Autodesk Inventor part; units mm, degrees
ref_plane "YZ Plane" through (0, 0, 0) normal (1, 0, 0) x (0, 1, 0)
ref_plane "XZ Plane" through (0, 0, 0) normal (0, 1, 0) x (-1, 0, 0)
ref_plane "XY Plane" through (0, 0, 0) normal (0, 0, 1) x (1, 0, 0)
sketch "Esquisse6" plane through (20, 29, 11.5) normal (-1, 0, 0) x (0, 0, 1)
  line L0 (0, -22) -> (-23, -22) construction
  line L1 (-23, -30.3566) -> (-23, -22) construction
  line L2 (0, -30.3566) -> (-23, -30.3566) construction
  line L3 (0, -30.3566) -> (0, -22) construction
  line L4 (-23, 0) -> (0, 0) construction
  line L5 (0, 8.3566) -> (0, 0) construction
  line L6 (-23, 8.3566) -> (0, 8.3566) construction
  line L7 (-23, 8.3566) -> (-23, 0) construction
  line L8 (-23, 8.3566) -> (-23, 0) construction
  line L9 (0, 8.3566) -> (-23, 8.3566) construction
  line L10 (0, 8.3566) -> (0, 0) construction
  line L11 (0, 8.3566) -> (0, 0) construction
  line L12 (-23, -30.3566) -> (-22, -27.6783)
  line L13 (-22, -27.6783) -> (-21, -27.6783)
  line L14 (-21, -27.6783) -> (-21, -24.6783)
  line L15 (-21, -24.6783) -> (-22, -24.6783)
  line L16 (-22, -24.6783) -> (-23, -22)
  line L17 (-23, -30.3566) -> (-23, -22) construction
  line L18 (-23, -26.1783) -> (-21, -26.1783) construction
  line L19 (-23, -22) -> (-23, -30.3566)
  line L20 (-23, -30.3566) -> (0, -30.3566)
  line L21 (-11.5, -22) -> (-11.5, -30.3566) construction
  line L22 (-23, -22) -> (0, -22) construction
  line L23 (0, -30.3566) -> (0, -22) construction
  line L24 (-23, -30.3566) -> (0, -30.3566) construction
  line L25 (0, -30.3566) -> (-1, -27.6783)
  line L26 (-1, -27.6783) -> (-2, -27.6783)
  line L27 (-2, -27.6783) -> (-2, -24.6783)
  line L28 (-2, -24.6783) -> (-1, -24.6783)
  line L29 (-1, -24.6783) -> (0, -22)
  line L30 (0, -30.3566) -> (0, -22) construction
  line L31 (0, -26.1783) -> (-2, -26.1783) construction
  line L32 (0, -22) -> (0, -30.3566)
  line L33 (0, -30.3566) -> (-23, -30.3566)
  dimension "d31" = 1
  dimension "d32" = 1
  dimension "d33" = 3
sketch "Esquisse1" plane through (0, 0, 0) normal (0, 1, 0) x (-1, 0, 0)
  arc A0 (0, -11.5) -> (0, 11.5) centre (0, 0) ccw
  line L0 (0, 11.5) -> (-20, 11.5)
  line L1 (-20, 11.5) -> (-20, -11.5)
  line L2 (-20, -11.5) -> (0, -11.5)
  dimension "d0" = 23
  dimension "d1" = 20
  dimension "d2" = 11.5
extrude "Plaque1" add sketch "Esquisse1" along normal blind 3
sketch "Esquisse2" plane through (0, 0, 0) normal (0, -1, 0) x (1, 0, 0)
  arc A0 (0, 11.5) -> (0, -11.5) centre (0, 0) ccw construction
  line L0 (0, 0) -> (-6, 0) construction
  point P0 (0, 6)
  point P1 (0, -6)
  point P2 (6, 0)
  dimension "d6" = 360
  dimension "d8" = 6
hole "Perçage1" at (0, 0, 0) at (0, 0, 6) at (-6, 0, 0) at (0, 0, -6) at (6, 0, 0) direction (0, 1, 0) diameter 4.05 end through all counterbore diameter 5.5 counterbore depth 1
ref_plane "Plan de construction1" through (0, 18, 0) normal (0, 1, 0) x (1, 0, 0)
mirror "Symétrie1" about plane through (0, 18, 0) normal (0, 1, 0)
sketch "Esquisse3" plane through (20, 0, 11.5) normal (1, 0, 0) x (0, 0, -1)
  line L0 (23, 3) -> (0, 3)
  line L1 (0, 0) -> (0, 3)
  line L2 (23, 0) -> (0, 0)
  line L3 (23, 0) -> (23, 3)
  line L4 (23, 33) -> (0, 33)
  line L5 (23, 36) -> (23, 33)
  line L6 (23, 36) -> (0, 36)
  line L7 (0, 36) -> (0, 33)
  line L8 (0, 0) -> (23, 0)
  line L9 (23, 0) -> (23, 36)
  line L10 (23, 36) -> (0, 36)
  line L11 (0, 36) -> (0, 0)
  point P0 (11.5, 0)
sheet face with bend "Face2" sketch "Esquisse3" thickness 3 toward (1, 0, 0) bend radius 4 contours L0 L11 L4 L9
bend "Pli1"
sketch "Esquisse4" plane through (23, 0, 11.5) normal (1, 0, 0) x (0, 0, -1)
  line L0 (23, 7) -> (0, 7) construction
  line L1 (23, 29) -> (23, 7) construction
  line L2 (0, 29) -> (23, 29) construction
  line L3 (0, 7) -> (0, 29) construction
  line L4 (23, 18) -> (0, 18) construction
  circle A0 centre (16.5, 23) radius 1.5
  line L5 (11.5, 18) -> (11.5, 7) construction
  circle A1 centre (16.5, 13) radius 1.5
  circle A2 centre (6.5, 23) radius 1.5
  circle A3 centre (6.5, 13) radius 1.5
  point P0 (11.5, 0)
  dimension "d22" = 10
  dimension "d23" = 3
  dimension "d25" = 10
extrude "Couper1" cut sketch "Esquisse4" against normal blind 3
equation "\"d2\" = 0.5 * d0"
equation "\"d9\" = ollo_hole"
equation "\"d11\" = ollo_ring"
equation "\"d12\" = ollo_depth"
equation "\"d14\" = Epaisseur"
equation "\"d25\" = d22"
equation "\"d26\" = Epaisseur"
equation "\"d17\" = RayonPli"
equation "\"d18\" = LargeurGrugeage"
equation "\"d20\" = RestesMinimum"
equation "\"d19\" = ProfondeurGrugeage"
equation "\"d21\" = RayonPli"
equation "\"LargeurGrugeage\" = Epaisseur"
equation "\"ProfondeurGrugeage\" = 0.5 * Epaisseur"
equation "\"TailleGrugeage\" = 4 * Epaisseur"
equation "\"RestesMinimum\" = 2 * Epaisseur"
equation "\"Rayondetransition\" = RayonPli"
equation "\"TailleRayonJacobi\" = RayonPli"
equation "\"TailleJeu\" = Epaisseur"
equation "\"d3\" = RayonPli"
properties part number "u" material "Plastique PMMA"
CAD build for the part. Positions are in the model's coordinates, mm. A direction names the side the tool comes from. Round coordinates to 2 decimals unless told otherwise and drop trailing zeros. Write each loop counter-clockwise with the first axis right and the second up, starting at its lowest first coordinate (ties: lowest second). Pieces come first, ordered by that corner, then holes.
(1) 3-axis set-ups, long thin cutter, end or side, ignore diameter. For faces 5 (the face through (-2.685, 35.493, 0.596)), 6 (the face through (2, 1, -5)), 7 (the face through (18.859, 4.203, -0.161)): which of +Z, -Z, +X, -X, +Y, -Y reach the whole face in a straight line?
(2) Slice it at B-B, the plane x = 10. Write the cut outline in (y, z), and give its area (3 significant figures).
(3) Drop flat-ended pins along their axis: P1, Ø2, axis at y = 10, z = 9, coming from the -X side; P2, Ø4, axis at x = 11, z = 4.5, coming from the -Y side; P3, Ø1.6, axis at x = 0.5, z = 6, coming from the -Y side. Give the stop position or say it passes through.
(4) Slice it at A-A, the plane y = 13. Write the cut outline in (x, z), and give its area (3 significant figures).
(5) Slice it at D-D, the plane z = 0. Count the separate pieces of the cut face and the enclosed holes in it, and give its area (3 significant figures).
(6) Probe line 1 along Z through (x, y) = (0, 33.65) (3 decimals); line 2 along Y through (x, z) = (13, 6.25); line 3 along Z through (x, y) = (6, 2.1) (3 decimals). List the from-to ranges inside material, lowest first.
(7) Mould opens along X. For faces 1 (the face through (21, 33.9, 0.2)), 2 (the face through (4.023, 33.986, 0.439)), 3 (the face through (-1.977, 33.986, 0.439)), 4 (the face through (21, 17, -11.5)) say: pulls with the +X half, pulls with the -X half, needs draft (parallel to the pull), parting line crosses it, or undercut.
(8) Slice it at C-C, the plane x = -5. Write the cut outline in (y, z), and give its area (3 significant figures).
From the geometry:
1. face 5: +Y
1. face 6: -Y
1. face 7: +Z, -Z, -X
2. outline: (0, -11.5) - (3, -11.5) - (3, 11.5) - (0, 11.5) - close; (33, -11.5) - (36, -11.5) - (36, 11.5) - (33, 11.5) - close
2. area: 138 mm2
3. P1: stops at x = 20
3. P2: stops at y = 0
3. P3: passes through
4. outline: (20, -11.5) - (23, -11.5) - (23, -6.5) - (20, -6.5) - close; (20, -3.5) - (23, -3.5) - (23, 3.5) - (20, 3.5) - close; (20, 6.5) - (23, 6.5) - (23, 11.5) - (20, 11.5) - close
4. area: 51.0 mm2
5. separate pieces: 7
5. enclosed holes: 0
5. area: 201 mm2
6. line 1: z = -11.5 to -8.025, -3.975 to -2.025, 2.025 to 3.975, 8.025 to 11.5
6. line 2: y = 0 to 3, 33 to 36
6. line 3: z = -11.5 to -2.025, 2.025 to 11.5
7. face 1: pulls with the +X half
7. face 2: undercut
7. face 3: undercut
7. face 4: needs draft
8. outline: (0, -10.36) - (3, -10.36) - (3, -1.76) - (1, -1.76) - (1, -2.56) - (0, -2.56) - close; (0, 2.56) - (1, 2.56) - (1, 1.76) - (3, 1.76) - (3, 10.36) - (0, 10.36) - close; (33, -10.36) - (36, -10.36) - (36, -2.56) - (35, -2.56) - (35, -1.76) - (33, -1.76) - close; (33, 1.76) - (35, 1.76) - (35, 2.56) - (36, 2.56) - (36, 10.36) - (33, 10.36) - close
8. area: 99.9 mm2
